Here's how the part is built. I have some questions about the finished solid (model axes, mm). Give positions to 0.01 mm unless a question says otherwise; leave off trailing zeros. Write each loop counter-clockwise with the first axis right and the second up, starting at its lowest first coordinate (ties: lowest second). Pieces come first, ordered by that corner, then holes. Notation, with made-up numbers: (60, 54.25) - (80, 54.25) arc R21 ccw to (80, 78.25) - close; hole circle Ø9 at (-13.75, 51.5). An arc over 180 degrees is marked (long way). Use one line per item in the form item = value. Start each with the question number.
from build123d import *

# Parameters (mm, degrees)
SKETCH_1_R      = 4
SKETCH_1_R_2    = 2
EXTRUDE_1_DEPTH = 3
SKETCH_2_R      = 5
SKETCH_2_R_2    = 2
EXTRUDE_2_DEPTH = 0.6
SKETCH_3_R      = 4
SKETCH_3_R_2    = 2
EXTRUDE_3_DEPTH = 1


with BuildPart() as part:
    # 草图1 → 凸台-拉伸1 (new body)
    with BuildSketch(Plane(origin=(0, 0, 0), x_dir=(1, 0, 0), z_dir=(0, 1, 0))):
        with Locations(Location((0, 0, 0), (0, 0, 270))):
            Circle(SKETCH_1_R)
        with Locations(Location((0, 0, 0), (0, 0, 270))):
            Circle(SKETCH_1_R_2, mode=Mode.SUBTRACT)
    extrude(amount=EXTRUDE_1_DEPTH)

    # 草图2 → 凸台-拉伸2 (add)
    with BuildSketch(Plane.XZ):
        with Locations(Location((0, 0, 0), (0, 0, 270))):
            Circle(SKETCH_2_R)
        with Locations(Location((0, 0, 0), (0, 0, 90))):
            Circle(SKETCH_2_R_2, mode=Mode.SUBTRACT)
    extrude(amount=-EXTRUDE_2_DEPTH)

    # 草图3 → 凸台-拉伸3 (add)
    with BuildSketch(Plane(origin=(0, 3, 0), x_dir=(1, 0, 0), z_dir=(0, 1, 0))):
        with Locations(Location((0, 0, 0), (0, 0, 90))):
            Circle(SKETCH_3_R)
        with Locations(Location((0, 0, 0), (0, 0, 270))):
            Circle(SKETCH_3_R_2, mode=Mode.SUBTRACT)
    extrude(amount=EXTRUDE_3_DEPTH)


solid = part.part
1. I want a section at A-A, the plane z = 0. List the corners of the cut face in (x, y) for me.
2. Please list where these lines run through material, in increasing order: line 1 (X direction, y = 1.65, z = 0); line 2 (Y direction, x = 3.5, z = 3); line 3 (Z direction, x = 0.5, y = 0.7).
3. I want a section at C-C, the plane x = 2.5. List the corners of the cut face in (y, z) for me.
4. I want a section at B-B, the plane x = 0. List the corners of the cut face in (y, z) for me.
5. I want a section at D-D, the plane y = 2.4. List the corners of the cut face in (x, z) for me.
6. For P1, Ø5, axis at x = 1, z = -1, coming from the +Y side; P2, Ø1, axis at y = 2.5, z = -1, coming from the +X side, each with a flat end and sliding along its axis, tell me the tip position at first contact or that it passes through.
Result sheet:
q1.outline = (-5, 0) - (-2, 0) - (-2, 4) - (-4, 4) - (-4, 0.6) - (-5, 0.6) - close; (2, 0) - (5, 0) - (5, 0.6) - (4, 0.6) - (4, 4) - (2, 4) - close
q2.line_1 = -4 to -2, 2 to 4
q2.line_2 = 0 to 0.6
q2.line_3 = -3.97 to -1.94, 1.94 to 3.97
q3.outline = (0, -4.33) - (0.6, -4.33) - (0.6, -3.12) - (4, -3.12) - (4, 3.12) - (0.6, 3.12) - (0.6, 4.33) - (0, 4.33) - close
q4.outline = (0, -5) - (0.6, -5) - (0.6, -4) - (4, -4) - (4, -2) - (0, -2) - close; (0, 2) - (4, 2) - (4, 4) - (0.6, 4) - (0.6, 5) - (0, 5) - close
q5.outline = circle Ø8 at (0, 0); hole circle Ø4 at (0, 0)
q6.P1 = 4
q6.P2 = 3.97
